Can you work these out from the model? Positions are in its coordinate system, mm. Face numbers are marked on the shaded views. Round coordinates to 2 decimals unless told otherwise and drop trailing zeros. Loops run counter-clockwise (first coordinate to the right, second up) from the corner with the lowest first, then second, coordinate; pieces in that order, holes last. Notation, with made-up numbers: (3.5, -28) -> (18.5, -28) arc R19 cw to (18.5, -7) -> close; hole circle Ø1 at (32.25, 49.25). An arc over 180 degrees is marked (long way). Answer as a JSON object with one key per item and string values.
```python
from build123d import *

# Parameters (mm, degrees)
BOSS_EXTRUDE1_DEPTH      = 2
BOSS_EXTRUDE1_DEPTH_BACK = 2
SKETCH2_R                = 2.5
SKETCH3_OUTSIDE_W        = 41.334
SKETCH3_OUTSIDE_H        = 42.572
SKETCH3_OUTSIDE_R        = 3.9
CUT_EXTRUDE1_DEPTH       = 8.302967433
CUT_EXTRUDE1_DRAFT       = -60
FILLET1_R                = 0.2
MIRROR1_COPY_1_SKETCH_W  = 41.334
MIRROR1_COPY_1_SKETCH_H  = 42.572
MIRROR1_COPY_1_SKETCH_R  = 3.9
MIRROR1_COPY_1_DEPTH     = 8.302967433
MIRROR1_COPY_1_DRAFT     = -60


with BuildPart() as part:
    # Sketch2 → Boss-Extrude1 (new, two sides: drawn at the far end of the back side and taken through both)
    with BuildSketch(Plane.XY.offset(-BOSS_EXTRUDE1_DEPTH_BACK)):
        Polygon((0, 4.618802154), (-4, 2.309401077), (-4, -2.309401077), (0, -4.618802154), (4, -2.309401077), (4, 2.309401077), align=None)
        Circle(SKETCH2_R, mode=Mode.SUBTRACT)
    extrude(amount=BOSS_EXTRUDE1_DEPTH + BOSS_EXTRUDE1_DEPTH_BACK)


with BuildPart() as cut_extrude1_tool:
    # Sketch3 outside → Cut-Extrude1 (with draft: the straight prism first)
    with BuildSketch(Plane.XY.offset(2)):
        Rectangle(SKETCH3_OUTSIDE_W, SKETCH3_OUTSIDE_H)
        Circle(SKETCH3_OUTSIDE_R, mode=Mode.SUBTRACT)
    extrude(amount=-CUT_EXTRUDE1_DEPTH)
    # Cut-Extrude1: the draft: its side faces are tilted about the plane it starts from
    cut_extrude1_sides = [cut_extrude1_tool.faces().sort_by_distance(p)[0] for p in [
        (0, -21.286, -2.151483717),
        (20.667, 0, -2.151483717),
        (0, 21.286, -2.151483717),
        (-20.667, 0, -2.151483717),
        (-3.9, 0, -2.151483717),
    ]]
    draft(cut_extrude1_sides, Plane.XY.offset(2), CUT_EXTRUDE1_DRAFT)


with BuildPart() as part_1:
    add(part.part)

    # Cut-Extrude1: cut by cut_extrude1_tool
    add(cut_extrude1_tool.part, mode=Mode.SUBTRACT)

    # Fillet1
    fillet1_edges = [part_1.edges().sort_by_distance(p)[0] for p in [
        (4, -2.309401077, -0.207500308),
        (0, -4.618802154, -0.207500308),
        (-4, -2.309401077, -0.207500308),
        (-4, 2.309401077, -0.207500308),
        (4, 2.309401077, -0.207500308),
        (0, 4.618802154, -0.207500308),
    ]]
    fillet(fillet1_edges, radius=FILLET1_R)

    # Cut-Extrude4 cone 1 section (through the dimple's axis) → Cut-Extrude4 (revolve, cut)
    with BuildSketch(Plane(origin=(0, 0, 2), x_dir=(0, -1, 0), z_dir=(1, 0, 0))):
        Polygon((0, 0), (2.63660254, 0), (0, 2.63660254), align=None)
    cut_extrude4 = revolve(axis=Axis((0, 0, 2), (0, 0, -1)), mode=Mode.SUBTRACT)

    # Mirror1: Cut-Extrude4 across plane
    add(cut_extrude4.mirror(Plane.XY), mode=Mode.SUBTRACT)


with BuildPart() as mirror1_copy_1_tool:
    # Mirror1 copy 1 sketch → Mirror1 copy 1 (with draft: the straight prism first)
    with BuildSketch(Plane(origin=(0, 0, -2), x_dir=(1, 0, 0), z_dir=(0, 0, -1))):
        Rectangle(MIRROR1_COPY_1_SKETCH_W, MIRROR1_COPY_1_SKETCH_H)
        Circle(MIRROR1_COPY_1_SKETCH_R, mode=Mode.SUBTRACT)
    extrude(amount=-MIRROR1_COPY_1_DEPTH)
    # Mirror1 copy 1: the draft: its side faces are tilted about the plane it starts from
    mirror1_copy_1_sides = [mirror1_copy_1_tool.faces().sort_by_distance(p)[0] for p in [
        (0, -21.286, 2.151483717),
        (20.667, 0, 2.151483717),
        (0, 21.286, 2.151483717),
        (-20.667, 0, 2.151483717),
        (-3.9, 0, 2.151483717),
    ]]
    draft(mirror1_copy_1_sides, Plane(origin=(0, 0, -2), x_dir=(1, 0, 0), z_dir=(0, 0, -1)), MIRROR1_COPY_1_DRAFT)


with BuildPart() as part_2:
    add(part_1.part)

    # Mirror1 copy 1: cut by mirror1_copy_1_tool
    add(mirror1_copy_1_tool.part, mode=Mode.SUBTRACT)


solid = part_2.part
```
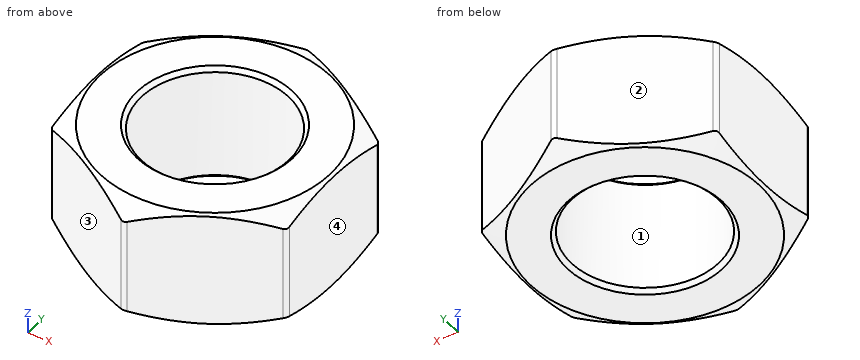
Q1. I want a section at A-A, the plane z = -0.45. Write out the boundary of the cut face in (x, y).
Determined:
{"outline": "(-4, -2.19) arc R0.2 ccw to (-3.9, -2.37) -> (-0.1, -4.56) arc R0.2 ccw to (0.1, -4.56) -> (3.9, -2.37) arc R0.2 ccw to (4, -2.19) -> (4, 2.19) arc R0.2 ccw to (3.9, 2.37) -> (0.1, 4.56) arc R0.2 ccw to (-0.1, 4.56) -> (-3.9, 2.37) arc R0.2 ccw to (-4, 2.19) -> close; hole circle Ø5 at (0, 0)"}
Q2. I'm going to push flat-ended pins straight in: pin 1 (4 mm diameter, centred on x = 0, y = 0, fed in from +Z); pin 2 (1.5 mm diameter, centred on x = 1, z = -1, fed in from -Y). Where does each tip first touch, or does it pass through?
Determined:
{"pin 1": "through", "pin 2": "y = -4.47"}
Q3. We'd pull the mould along Y, two halves only. Please class the marked faces 1, 2, 3 and 4: pulls with the +Y half, pulls with the -Y half, needs draft (parallel to the pull), parting line crosses it, or undercut.
Determined:
{"face 1": "undercut", "face 2": "pulls with the +Y half", "face 3": "pulls with the -Y half", "face 4": "needs draft"}
Q4. If I drill on L1, parallel to Y at x = 0, z = -0.35; L2, parallel to X at y = 0, z = -0.9; L3, parallel to X at y = 1.75, z = -1.1, over which ranges is the centre line in solid material (lowest first)? Write a range as [from, to].
Determined:
{"L1": "[-4.59, -2.5], [2.5, 4.59]", "L2": "[-4, -2.5], [2.5, 4]", "L3": "[-4, -1.79], [1.79, 4]"}
Q5. I want a section at B-B, the plane y = 0. Write out the boundary of the cut face in (x, z).
Determined:
{"outline": "(-4, -1.94) -> (-3.9, -2) -> (-2.64, -2) -> (-2.5, -1.86) -> (-2.5, 1.86) -> (-2.64, 2) -> (-3.9, 2) -> (-4, 1.94) -> close; (2.5, -1.86) -> (2.64, -2) -> (3.9, -2) -> (4, -1.94) -> (4, 1.94) -> (3.9, 2) -> (2.64, 2) -> (2.5, 1.86) -> close"}
